Build history of the part. All positions in model axes, mm. Round coordinates to 2 decimals unless told otherwise and drop trailing zeros. Order: outer loops, then holes, each group sorted by start corner. A loop starts at its lowest first (then second) coordinate and runs counter-clockwise, first axis right, second up. Notation, with made-up numbers: (-40, 15.25) -> (-5, 15.25) arc R17 ccw to (-5, 38.25) -> close; hole circle Ø11 at (-25, 23). An arc over 180 degrees is marked (long way). Answer as CSV lines item,"result". Start each with the question number.
```python
from build123d import *

# Parameters (mm, degrees)
SKETCH1_W               = 254
SKETCH1_H               = 152.4
SKETCH1_W_2             = 6.35
SKETCH1_H_2             = 139.7
SKETCH1_W_3             = 3.175
SKETCH1_W_4             = 100.0125
SKETCH1_H_3             = 6.34492
BOSS_EXTRUDE1_DEPTH     = 6.35
SKETCH2_W               = 209.55
SKETCH2_H               = 114.3
CUT_EXTRUDE1_DEPTH      = 65.278
CUT_EXTRUDE1_DEPTH_BACK = 127


with BuildPart() as part:
    # Sketch1 → Boss-Extrude1 (new body)
    with BuildSketch(Plane(origin=(0, 0, 0), x_dir=(1, 0, 0), z_dir=(0, 1, 0))):
        Rectangle(SKETCH1_W, SKETCH1_H)
        with Locations((117.475, 0)):
            Rectangle(SKETCH1_W_2, SKETCH1_H_2, mode=Mode.SUBTRACT)
        Rectangle(SKETCH1_W_3, SKETCH1_H_2, mode=Mode.SUBTRACT)
        with Locations((-117.475, 0)):
            Rectangle(SKETCH1_W_2, SKETCH1_H_2, mode=Mode.SUBTRACT)
        with Locations((-57.94375, 66.67754)):
            Rectangle(SKETCH1_W_4, SKETCH1_H_3, mode=Mode.SUBTRACT)
        with Locations((57.94375, -66.68262)):
            Rectangle(SKETCH1_W_4, SKETCH1_H_3, mode=Mode.SUBTRACT)
        with Locations((57.94375, 66.67754)):
            Rectangle(SKETCH1_W_4, SKETCH1_H_3, mode=Mode.SUBTRACT)
        with Locations((-57.94375, -66.67754)):
            Rectangle(SKETCH1_W_4, SKETCH1_H_3, mode=Mode.SUBTRACT)
    extrude(amount=BOSS_EXTRUDE1_DEPTH)

    # Sketch2 → Cut-Extrude1 (cut, two sides)
    with BuildSketch(Plane(origin=(0, 0, 0), x_dir=(1, 0, 0), z_dir=(0, 1, 0))) as cut_extrude1_sk:
        Rectangle(SKETCH2_W, SKETCH2_H)
    extrude(amount=CUT_EXTRUDE1_DEPTH, mode=Mode.SUBTRACT)
    extrude(cut_extrude1_sk.sketch, amount=-CUT_EXTRUDE1_DEPTH_BACK, mode=Mode.SUBTRACT)


solid = part.part
```
Q1. Slice it at A-A, the plane z = 22. Write the cut outline in (x, y) (3 decimals), plus the area to 3 significant figures.
Q2. Probe L1, parallel to X at y = 4.25, z = -67; L2, parallel to Z at x = -69.5, y = 2; L3, parallel to X at y = 5, z = -52.5 (3 decimals). List the from-to ranges inside material, lowest first.
Q3. Two-plate mould, pull along X, no slides. Class faces 1 (the face through (-19, 6.35, -62)), 2 (the face through (57, 3, -63.505)): +X half, -X half, draft (parallel to the pull), parting line (faces both ways), or undercut.
Q4. Slice it at C-C, the plane y = 2.25. Count the separate pieces of the cut face and the enclosed holes in it, plus the area to 3 significant figures.
Q5. Flat gauge pin, fed straight in: pin 1 Ø8 at (x, z) = (-52, 51.5) entering from -Y. Where does the tip first touch, or does it go through?
Q6. Slice it at B-B, the plane x = -51.5. Write the cut outline in (y, z).
Solutions:
1,outline,"(-127, 0) -> (-120.65, 0) -> (-120.65, 6.35) -> (-127, 6.35) -> close; (-114.3, 0) -> (-104.775, 0) -> (-104.775, 6.35) -> (-114.3, 6.35) -> close; (104.775, 0) -> (114.3, 0) -> (114.3, 6.35) -> (104.775, 6.35) -> close; (120.65, 0) -> (127, 0) -> (127, 6.35) -> (120.65, 6.35) -> close"
1,area,"202 mm2"
2,L1,"x = -127 to -120.65, -114.3 to -107.95, -7.94 to -1.59, 1.59 to 7.94, 107.95 to 114.3, 120.65 to 127"
2,L2,"z = -76.2 to -69.85, -63.51 to -57.15, 57.15 to 63.51, 69.85 to 76.2"
2,L3,"x = -127 to -120.65, -114.3 to -104.775, 104.775 to 114.3, 120.65 to 127"
3,face 1,"draft"
3,face 2,"undercut"
4,separate pieces,"1"
4,enclosed holes,"7"
4,area,"10,400 mm2"
5,pin 1,"passes through"
6,outline,"(0, -76.2) -> (6.35, -76.2) -> (6.35, -69.85) -> (0, -69.85) -> close; (0, -63.51) -> (6.35, -63.51) -> (6.35, -57.15) -> (0, -57.15) -> close; (0, 57.15) -> (6.35, 57.15) -> (6.35, 63.51) -> (0, 63.51) -> close; (0, 69.85) -> (6.35, 69.85) -> (6.35, 76.2) -> (0, 76.2) -> close"
